Autodesk Inventor part; units mm, degrees
ref_plane "YZ Plane" through (0, 0, 0) normal (1, 0, 0) x (0, 1, 0)
ref_plane "XZ Plane" through (0, 0, 0) normal (0, 1, 0) x (-1, 0, 0)
ref_plane "XY Plane" through (0, 0, 0) normal (0, 0, 1) x (1, 0, 0)
sketch "草图1" plane through (0, 0, 0) normal (0, 1, 0) x (-1, 0, 0)
  line L0 (0, 0) -> (27, 0)
  line L1 (27, 0) -> (27, -56)
  line L2 (27, -56) -> (0, -56)
  line L3 (0, -56) -> (0, 0)
  dimension "d0" = 27
  dimension "d1" = 56
extrude "拉伸1" add sketch "草图1" along normal blind 3
sketch "草图2" plane through (0, 0, 0) normal (1, 0, 0) x (0, 0, -1)
  line L0 (56, 3) -> (0, 3)
  line L1 (28, 3) -> (28, -4.4631)
  line L2 (19.0299, 3) -> (19.0299, 2.5)
  line L3 (28, 2.5) -> (2, 2.5)
  line L4 (2, 2.5) -> (2, 0.5)
  line L5 (2, 0.5) -> (28, 0.5)
  line L6 (28, 0.5) -> (28, 2.5)
  point P0 (0, 0)
  dimension "d4" = 0.5
  dimension "d5" = 26
  dimension "d6" = 2
extrude "拉伸2" cut sketch "草图2" against normal blind 25 contours L1 L5 L4 L3
mirror "镜像1" about plane through (0, 2.5, -28) normal (0, 0, 1) of "拉伸2"
sketch "草图3" plane through (0, 0, 0) normal (1, 0, 0) x (0, 0, -1)
  point P0 (0, 0)
sketch "草图4" plane through (0, 0, 0) normal (1, 0, 0) x (0, 0, -1)
  line L0 (56, 3) -> (0, 3)
  line L1 (28, 3) -> (28, -1.1507)
  line L2 (28, 3) -> (3, 3)
  line L3 (3, 3) -> (3, 2.5)
  line L4 (54, 2.5) -> (2, 2.5)
  line L5 (0, 0) -> (56, 0)
  line L6 (56, 0) -> (56, 3)
  line L7 (0, 3) -> (56, 3)
  line L8 (0, 0) -> (0, 3)
  line L9 (2, 2.5) -> (54, 2.5)
  line L10 (54, 2.5) -> (54, 0.5)
  line L11 (54, 0.5) -> (2, 0.5)
  line L12 (2, 0.5) -> (2, 2.5)
  point P0 (28, 2.5)
  dimension "d9" = 25
extrude "拉伸3" cut sketch "草图4" against normal blind 25 contours L1 L4 L3 L0
mirror "镜像2" about plane through (0, 3, -28) normal (0, 0, 1) of "拉伸3"
Could you check a few things on this model? Use its own coordinates, in mm. A direction names the side the tool comes from. Coordinates: 2 decimals unless noted, no trailing zeros. Loops run counter-clockwise (first coordinate to the right, second up) from the corner with the lowest first, then second, coordinate; pieces in that order, holes last.
1. Imagine slicing it at B-B (x = -18.75). Please give me the cut outline in (y, z), and give its area (3 significant figures).
2. Imagine slicing it at C-C (z = -4). Please give me the cut outline in (x, y), and give its area (3 significant figures).
3. I need wall thicknesses on L1, parallel to Z at x = -9.25, y = 1.9; L2, parallel to Z at x = -1.5, y = 2.9; L3, parallel to X at y = 2.6, z = -47. Which ranges of each line are inside material? Lowest first, please.
4. Imagine slicing it at A-A (y = 1.1). Please give me the cut outline in (x, z).
5. We'd pull the mould along Z, two halves only. Please class faces 1 (the face through (-12, 1, -54)), 2 (the face through (-14, 1, -56)), 3 (the face through (0, 0.2, -28.1)): released by +Z, released by -Z, zero draft, split by the parting line, or undercut.
6. For faces 4 (the face through (-12.3, 2.5, -2.5)), 5 (the face through (-25.4, 3, -23.7)), which set-ups out of +Z, -Z, +X, -X, +Y, -Y let a thin tool reach every point of the face, with its end or its side?
7. For P1, Ø1.5, axis at x = -13, y = 1.5, coming from the +Z side; P2, Ø3, axis at x = -21.5, z = -19.5, coming from the +Y side, each with a flat end and sliding along its axis, tell me the tip position at first contact or that it passes through.
Computed values:
1. outline: (0, -56) - (3, -56) - (3, -53) - (2.5, -53) - (2.5, -54) - (0.5, -54) - (0.5, -2) - (2.5, -2) - (2.5, -3) - (3, -3) - (3, 0) - (0, 0) - close
1. area: 39.0 mm2
2. outline: (-27, 0) - (0, 0) - (0, 0.5) - (-25, 0.5) - (-25, 3) - (-27, 3) - close
2. area: 18.5 mm2
3. L1: z = -56 to -54, -2 to 0
3. L2: z = -56 to -53, -3 to 0
3. L3: x = -27 to -25
4. outline: (-27, -56) - (0, -56) - (0, -54) - (-25, -54) - (-25, -2) - (0, -2) - (0, 0) - (-27, 0) - close
5. face 1: undercut
5. face 2: released by -Z
5. face 3: zero draft
6. face 4: +X
6. face 5: +Z, -Z, +X, -X, +Y
7. P1: stops at z = 0
7. P2: stops at y = 0.5
